The listing builds one solid part. Answer for the finished solid, in the listing's coordinates (mm). Round coordinates to 2 decimals unless told otherwise and drop trailing zeros. Order: outer loops, then holes, each group sorted by start corner. A loop starts at its lowest first (then second) coordinate and runs counter-clockwise, first axis right, second up. Notation, with made-up numbers: (84, 84.5) - (136, 84.5) arc R15 ccw to (136, 101.5) - close; hole circle Ø5 at (71, 67.5). An arc over 180 degrees is marked (long way). One line per item, written item: value. Start each with the question number.
1. Section B-B, the plane y = 1.8 is taken. Give the vertices of the cut face in (x, z), then the cut area to 3 significant figures.
2. A flat-ended cylindrical pin translates along its axis: P1, Ø2, axis at x = 52.5, y = -0.5, coming from the +Z side. Find the tip coordinate at first contact, or state that the pin passes through.
3. Straight lines are drawn through the part: line 1 (X direction, y = 1.5, z = 0); line 2 (X direction, y = 1.8, z = -51); line 3 (Z direction, x = 37, y = 0.7). For each, find the intervals that lie inside material, in ascending order.
4. Section A-A, the plane x = 0 is taken. Give the vertices of the cut face in (y, z), then the cut area to 3 significant figures.
5. Section C-C, the plane z = 0 is taken. Give the vertices of the cut face in (x, y), then the cut area to 3 significant figures.
from build123d import *

# Parameters (mm, degrees)
SKETCH_6_R      = 72.75
SKETCH_6_R_2    = 69.1
EXTRUDE_4_DEPTH = 2.4
SKETCH_6_3_R    = 65
EXTRUDE_5_DEPTH = 2.4
EXTRUDE_START   = -1
SKETCH_6_4_R    = 72.75
SKETCH_6_4_R_2  = 69.1
SKETCH_6_4_R_3  = 65
EXTRUDE_6_DEPTH = 1


with BuildPart() as part:
    # Sketch 6 → Extrude 4 (new body)
    with BuildSketch(Plane(origin=(0, 0, 0), x_dir=(1, 0, 0), z_dir=(0, 1, 0))):
        with Locations(Location((0, 0, 0), (0, 0, 270))):
            Circle(SKETCH_6_R)
        with Locations(Location((0, 0, 0), (0, 0, 270))):
            Circle(SKETCH_6_R_2, mode=Mode.SUBTRACT)
    extrude(amount=EXTRUDE_4_DEPTH)



with BuildPart() as body_2:
    # Sketch 6_3 → Extrude 5 (new body)
    with BuildSketch(Plane(origin=(0, 0, 0), x_dir=(1, 0, 0), z_dir=(0, 1, 0))):
        with Locations(Location((0, 0, 0), (0, 0, 270))):
            Circle(SKETCH_6_3_R)
    extrude(amount=EXTRUDE_5_DEPTH)


with BuildPart() as part_1:
    add(part.part)

    add(body_2.part)  # Extrude 6 merges body 2
    # Sketch 6_4 → Extrude 6 (add)
    # profile 1 of 3: a face of its own
    with BuildSketch(Plane(origin=(0, 0, 0), x_dir=(1, 0, 0), z_dir=(0, 1, 0)).offset(EXTRUDE_START)):
        with Locations(Location((0, 0, 0), (0, 0, 270))):
            Circle(SKETCH_6_4_R)
        with Locations(Location((0, 0, 0), (0, 0, 270))):
            Circle(SKETCH_6_4_R_2, mode=Mode.SUBTRACT)
    # profile 2 of 3: a face of its own
    with BuildSketch(Plane(origin=(0, 0, 0), x_dir=(1, 0, 0), z_dir=(0, 1, 0)).offset(EXTRUDE_START)):
        with Locations(Location((0, 0, 0), (0, 0, 270))):
            Circle(SKETCH_6_4_R_2)
        with Locations(Location((0, 0, 0), (0, 0, 270))):
            Circle(SKETCH_6_4_R_3, mode=Mode.SUBTRACT)
    # profile 3 of 3: a face of its own
    with BuildSketch(Plane(origin=(0, 0, 0), x_dir=(1, 0, 0), z_dir=(0, 1, 0)).offset(EXTRUDE_START)):
        with Locations(Location((0, 0, 0), (0, 0, 270))):
            Circle(SKETCH_6_4_R_3)
    extrude(amount=EXTRUDE_6_DEPTH)


solid = part_1.part
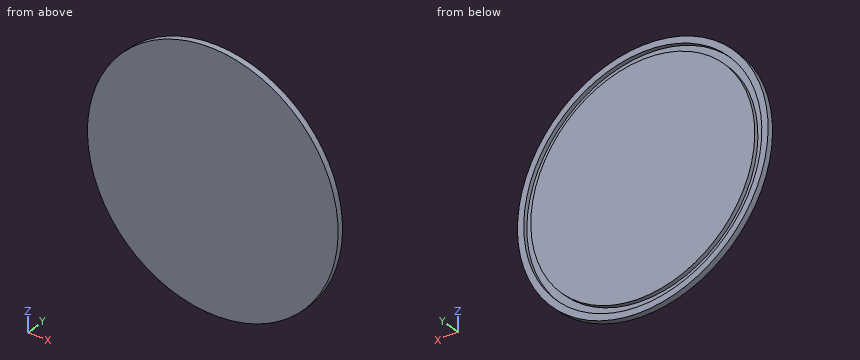
Answer list:
1. outline: circle Ø145.5 at (0, 0); circle Ø130 at (0, 0); hole circle Ø138.2 at (0, 0)
1. area: 14,900 mm²
2. P1: stops at z = 51.38
3. line 1: x = -72.75 to -69.1, -65 to 65, 69.1 to 72.75
3. line 2: x = -51.88 to -46.62, -40.3 to 40.3, 46.62 to 51.88
3. line 3: z = -62.64 to -58.36, -53.44 to 53.44, 58.36 to 62.64
4. outline: (-1, -72.75) - (2.4, -72.75) - (2.4, -69.1) - (0, -69.1) - (0, -65) - (2.4, -65) - (2.4, 65) - (0, 65) - (0, 69.1) - (2.4, 69.1) - (2.4, 72.75) - (-1, 72.75) - close
4. area: 475 mm²
5. outline: (-72.75, -1) - (72.75, -1) - (72.75, 2.4) - (69.1, 2.4) - (69.1, 0) - (65, 0) - (65, 2.4) - (-65, 2.4) - (-65, 0) - (-69.1, 0) - (-69.1, 2.4) - (-72.75, 2.4) - close
5. area: 475 mm²
